```python
from build123d import *

# Parameters (mm, degrees)
SKETCH_R     = 2
PAD_DEPTH    = 5
CHAMFER_SIZE = 1.5
FILLET_R     = 1


with BuildPart() as part:
    # Sketch → Pad (new body)
    with BuildSketch(Plane.XY):
        with BuildLine():
            ThreePointArc((0, 7.5), (-7.5, 0), (0, -7.5))
            Line((0, -7.5), (15, -7.5))
            ThreePointArc((15, -7.5), (22.5, 0), (15, 7.5))
            Line((0, 7.5), (15, 7.5))
        make_face()
        Circle(SKETCH_R, mode=Mode.SUBTRACT)
        with Locations((15, 0)):
            Circle(SKETCH_R, mode=Mode.SUBTRACT)
    extrude(amount=PAD_DEPTH)

    # Chamfer
    chamfer_edges = [part.edges().sort_by_distance(p)[0] for p in [
        (-2, 0, 5),
        (13, 0, 5),
    ]]
    chamfer(chamfer_edges, length=CHAMFER_SIZE)

    # Fillet
    fillet_edges = [part.edges().sort_by_distance(p)[0] for p in [
        (7.5, -7.5, 5),
    ]]
    fillet(fillet_edges, radius=FILLET_R)


solid = part.part
```
CAD build for the part. Positions are in the model's coordinates, mm. Coordinates: 2 decimals unless noted, no trailing zeros. Loops run counter-clockwise (first coordinate to the right, second up) from the corner with the lowest first, then second, coordinate; pieces in that order, holes last. Notation, with made-up numbers: (5, 46) - (22, 46) arc R22 cw to (22, 84) - close; hole circle Ø3 at (-11.5, 74). An arc over 180 degrees is marked (long way). Use CSV: the item, a comma, the result in double quotes. Start each with the question number.
Q1. Cut at B-B, the plane z = 2. List the corners of the cut face in (x, y), then the cut area to 3 significant figures.
Q2. Probe probe 1 along X at (y, z) = (-2, 4.65); probe 2 along Y at (x, z) = (15, 1.2); probe 3 along Y at (x, z) = (14.5, 4.6). List the from-to ranges inside material, lowest first. Write a range as from..to.
Q3. Two-plate mould, pull along X, no slides. Class faces 1 (the flat face through (7, 7.5, 2)), 2 (the cylindrical face through (0, -2, 2)), 3 (the cylindrical face through (22.5, -0.16, 1.97)): +X half, -X half, draft (parallel to the pull), parting line (faces both ways), or undercut.
Q4. Cut at A-A, the plane y = 0. List the corners of the cut face in (x, z), then the cut area to 3 significant figures.
Q5. Drop flat-ended pins along their axis: P1, Ø6.5, axis at x = 15, y = 0, coming from the +Z side; P2, Ø3, axis at y = -5, z = 3, coming from the +X side; P3, Ø1, axis at y = -5, z = 2, coming from the +X side. Give the stop position or say it passes through.
Here are the results:
1,outline,"(0, -7.5) - (15, -7.5) arc R7.5 ccw to (15, 7.5) - (0, 7.5) arc R7.5 ccw to start; hole circle Ø4 at (0, 0); hole circle Ø4 at (15, 0)"
1,area,"377 mm2"
2,probe 1,"-6.98..-2.43, 2.43..12.57, 17.43..21.98"
2,probe 2,"-7.5..-2, 2..7.5"
2,probe 3,"-7.3..-3.06, 3.06..7.3"
3,face 1,"draft"
3,face 2,"undercut"
3,face 3,"+X half"
4,outline,"(-7.5, 0) - (-2, 0) - (-2, 3.5) - (-3.5, 5) - (-6.5, 5) arc R1 ccw to (-7.5, 4) - close; (2, 0) - (13, 0) - (13, 3.5) - (11.5, 5) - (3.5, 5) - (2, 3.5) - close; (17, 0) - (22.5, 0) - (22.5, 4) arc R1 ccw to (21.5, 5) - (18.5, 5) - (17, 3.5) - close"
4,area,"105 mm2"
5,P1,"z = 4.75"
5,P2,"x = 21.63"
5,P3,"x = 21"
